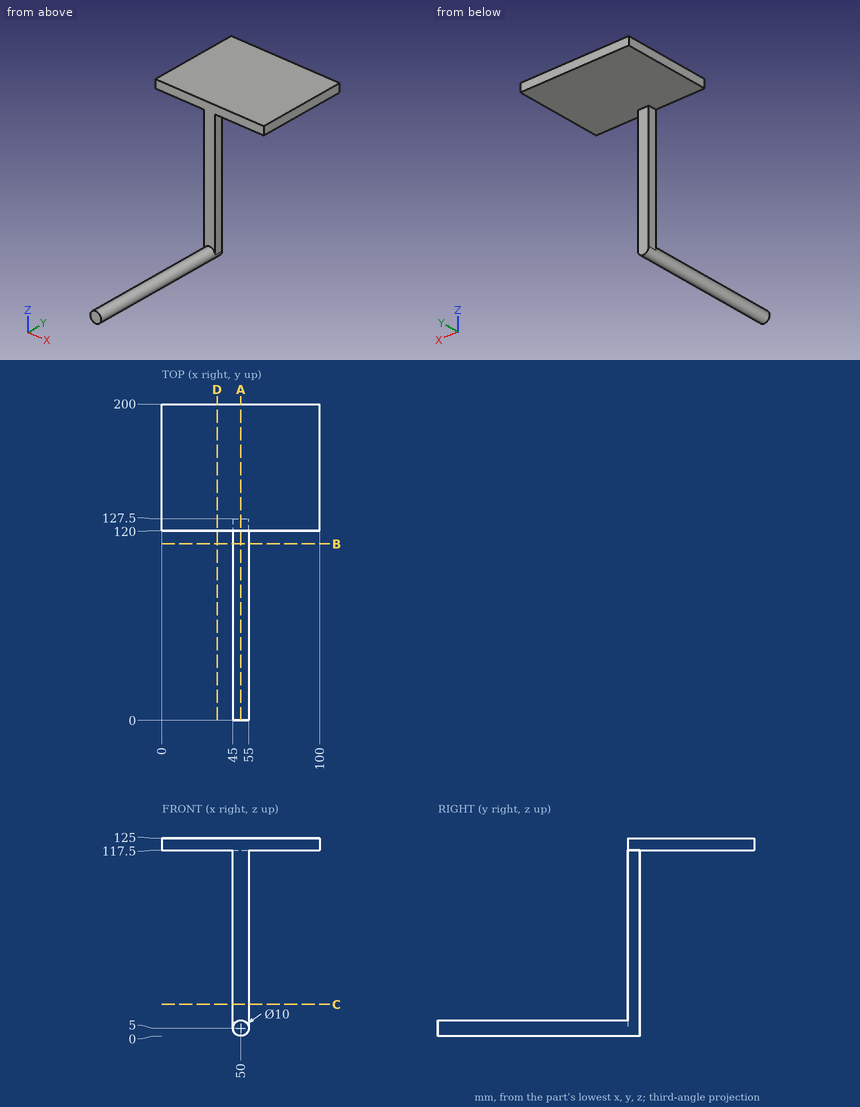
The drawing under review shows one solid part. Ordinate dimensions are in mm from its lowest x, y, z. Give positions to 0.01 mm unless a question says otherwise; leave off trailing zeros. Order: outer loops, then holes, each group sorted by start corner. A loop starts at its lowest first (then second) coordinate and runs counter-clockwise, first axis right, second up. Notation, with made-up numbers: M 78.25,33.5 L 111.25,33.5 A17 ccw 111.25,55.5 Z; hole C -36.5,71 d10. An arc over 180 degrees is marked long. Answer in a Markdown table with one row per item. Add a question column.
1. Add section B-B on y = 111.5. State the section outline as (x, z) points, plus the area to 3 significant figures.
2. Add section A-A on x = 50. State the section outline as (y, z) points.
3. Add section C-C on z = 20. State the section outline as (x, y) points.
4. Add section D-D on x = 35. State the section outline as (y, z) points.
5. For pin 1 Ø12 at (x, y) = (69, 175) entering from -Z; pin 2 Ø3 at (x, z) = (51, 61.5) entering from +Y; pin 3 Ø10 at (y, z) = (127.5, 51.5) entering from -X, all flat-tipped, find the tip position at first contact; note any pin that passes through.
6. To check wall thickness, follow line 1 along Z through (x, y) = (55, 154); line 2 along Y through (x, z) = (50, 34); line 3 along X through (y, z) = (28, 8). State the ranges of each line that lie inside material, in increasing order.
The answers:
| question | item | result |
|---|---|---|
| 1 | outline | C 50,5 d10 |
| 1 | area | 78.5 mm2 |
| 2 | outline | M 0,0 L 127.5,0 L 127.5,117.5 L 200,117.5 L 200,125 L 120,125 L 120,10 L 0,10 Z |
| 3 | outline | M 45,120 L 55,120 L 55,127.5 L 45,127.5 Z |
| 4 | outline | M 120,117.5 L 200,117.5 L 200,125 L 120,125 Z |
| 5 | pin 1 | z = 117.5 |
| 5 | pin 2 | y = 127.5 |
| 5 | pin 3 | x = 45 |
| 6 | line 1 | 117.5 to 125 |
| 6 | line 2 | 120 to 127.5 |
| 6 | line 3 | 46 to 54 |
